The model under review builds one solid part; all positions refer to its coordinate system, in mm. Round coordinates to 2 decimals unless told otherwise and drop trailing zeros. Write each loop counter-clockwise with the first axis right and the second up, starting at its lowest first coordinate (ties: lowest second). Pieces come first, ordered by that corner, then holes. Notation, with made-up numbers: (19.25, 78) - (30.25, 78) arc R13 cw to (30.25, 88) - close; hole circle Ø2 at (-34.5, -7). An arc over 180 degrees is marked (long way). One line per question, with ' | ' between items. Start each with the question number.
```python
from build123d import *

# Parameters (mm, degrees)
SKETCH020_W     = 6
SKETCH020_H     = 60
PAD004_DEPTH    = 31
SKETCH021_R     = 11.2
POCKET_DEPTH    = 6.001
SKETCH028_R     = 0.8
POCKET010_DEPTH = 15
POCKET011_DEPTH = 6.001
FILLET_R        = 1


with BuildPart() as part:
    # Sketch020 → Pad004 (new body)
    with BuildSketch(Plane.XY):
        with Locations((70, -5)):
            Rectangle(SKETCH020_W, SKETCH020_H)
    extrude(amount=PAD004_DEPTH)

    # Sketch021 → Pocket (cut, through all)
    with BuildSketch(Plane.YZ.offset(73)):
        with Locations((-5, 31)):
            Circle(SKETCH021_R)
    extrude(amount=-POCKET_DEPTH, mode=Mode.SUBTRACT)

    # Sketch028 → Pocket010 (cut)
    with BuildSketch(Plane.XY.offset(31)):
        with Locations((70, 9)):
            Circle(SKETCH028_R)
        with Locations((70, -19)):
            Circle(SKETCH028_R)
    extrude(amount=-POCKET010_DEPTH, mode=Mode.SUBTRACT)

    # Sketch029 → Pocket011 (cut, through all)
    with BuildSketch(Plane.YZ.offset(73)):
        Polygon((25, 3), (12.5, 32), (-22.5, 32), (-35, 3), (-38.294894757, 52.1665199783), (33.061305243, 52.1665199783), align=None)
    extrude(amount=-POCKET011_DEPTH, mode=Mode.SUBTRACT)

    # Fillet
    fillet_edges = [part.edges().sort_by_distance(p)[0] for p in [
        (73, 18.965517, 17),
        (70, 12.931034, 31),
        (67, 18.965517, 17),
        (70, 25, 3),
        (73, -28.965517, 17),
        (70, -35, 3),
        (67, -28.965517, 17),
        (70, -22.931034, 31),
    ]]
    fillet(fillet_edges, radius=FILLET_R)


solid = part.part
```
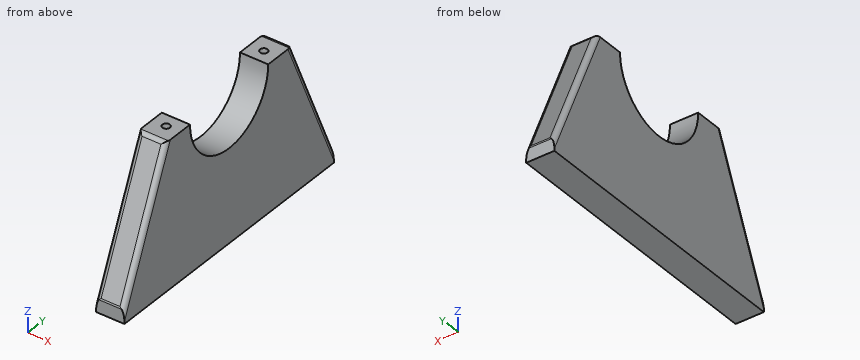
1. Add section C-C, the plane z = 29.5. State how many separate pieces and enclosed holes the cut face has, then the cut area to 3 significant figures.
2. Add section A-A, the plane x = 70. Write out the cut boundary in (y, z), then the cut area to 3 significant figures.
3. Wall thickness on line 1 along Y through (x, z) = (70, 21); line 2 along Y through (x, z) = (70, 19.5); line 3 along Y through (x, z) = (70, 27.25): over which ranges is each line inside the solid? List them lowest first. Write a range as [from, to].
4. Clearance check with a flat-ended pin moving along its axis: P1, Ø0.8, axis at x = 70, y = -19, coming from the +Z side. State where the tip first meets the part, or that it passes through.
5. Add section B-B, the plane y = 9. Write out the cut boundary in (x, z), then the cut area to 3 significant figures.
Geometry check:
1) separate pieces: 2 | enclosed holes: 2 | area: 84.8 mm2
2) outline: (-35, 0) - (25, 0) - (25, 2.79) arc R1 ccw to (24.92, 3.19) - (13.19, 30.4) arc R1 ccw to (12.27, 31) - (9.8, 31) - (9.8, 16) - (8.2, 16) - (8.2, 31) - (6.2, 31) arc R11.2 cw to (-16.2, 31) - (-18.2, 31) - (-18.2, 16) - (-19.8, 16) - (-19.8, 31) - (-22.27, 31) arc R1 ccw to (-23.19, 30.4) - (-34.92, 3.19) arc R1 ccw to (-35, 2.79) - close | area: 1,280 mm2
3) line 1: y = [-27.24, -19.8], [-18.2, -10.04], [0.04, 8.2], [9.8, 17.24] | line 2: y = [-27.89, -19.8], [-18.2, 8.2], [9.8, 17.89] | line 3: y = [-24.55, -19.8], [-18.2, -15.55], [5.55, 8.2], [9.8, 14.55]
4) P1: stops at z = 16
5) outline: (67, 0) - (73, 0) - (73, 31) - (70.8, 31) - (70.8, 16) - (69.2, 16) - (69.2, 31) - (67, 31) - close | area: 162 mm2
